```python
from build123d import *

# Parameters (mm, degrees)
SKETCH_1_R                         = 4
SKETCH_1_R_2                       = 1.5
SKETCH_1_R_3                       = 2
SM_BASE_FLANGE_1_DEPTH             = 2
SM_EDGE_FLANGE_1_STRIP_W           = 9.4732
SM_EDGE_FLANGE_1_STRIP_H           = 2
SM_EDGE_FLANGE_1_STRIP_CUT_DEPTH   = 9
SM_EDGE_FLANGE_1_STRIP_2_W         = 9.4732
SM_EDGE_FLANGE_1_STRIP_2_H         = 2
SM_EDGE_FLANGE_1_STRIP_CUT_2_DEPTH = 9
SM_EDGE_FLANGE_1_DEPTH             = 9
SM_EDGE_FLANGE_1_BEND_DEPTH        = 9
SM_EDGE_FLANGE_2_STRIP_W           = 9.4732
SM_EDGE_FLANGE_2_STRIP_H           = 2
SM_EDGE_FLANGE_2_STRIP_CUT_DEPTH   = 42
SM_EDGE_FLANGE_2_DEPTH             = 42
SKETCH_15_R                        = 1.5
CUT_EXTRUDE_1_DEPTH                = 10
SKETCH_16_R                        = 2
CUT_EXTRUDE_2_DEPTH                = 10
FILLET_1_R                         = 2


# Sheet-metal steps are written as plain solids
with BuildPart() as part:
    # Sketch 1 → 基体-法兰1 (new body)
    with BuildSketch(Plane.XY):
        Polygon((0, 0), (9, 0), (9, -6), (11, -6), (11, 4), (48, 4), (48, -6), (50, -6), (50, 0), (59, 0), (59, -25), (50.5, -25), (50.5, -33), (8.5, -33), (8.5, -25), (0, -25), align=None)
        with Locations((19, -8)):
            Circle(SKETCH_1_R, mode=Mode.SUBTRACT)
        with Locations((40, -8)):
            Circle(SKETCH_1_R, mode=Mode.SUBTRACT)
        with Locations((29.5, -19)):
            Circle(SKETCH_1_R, mode=Mode.SUBTRACT)
        with Locations((19, -1)):
            Circle(SKETCH_1_R_2, mode=Mode.SUBTRACT)
        with Locations((19, -15)):
            Circle(SKETCH_1_R_2, mode=Mode.SUBTRACT)
        with Locations((26, -8)):
            Circle(SKETCH_1_R_2, mode=Mode.SUBTRACT)
        with Locations((12, -8)):
            Circle(SKETCH_1_R_2, mode=Mode.SUBTRACT)
        with Locations(Location((33, -8, 0), (0, 0, 180))):
            Circle(SKETCH_1_R_2, mode=Mode.SUBTRACT)
        with Locations(Location((40, -15, 0), (0, 0, 180))):
            Circle(SKETCH_1_R_2, mode=Mode.SUBTRACT)
        with Locations(Location((47, -8, 0), (0, 0, 180))):
            Circle(SKETCH_1_R_2, mode=Mode.SUBTRACT)
        with Locations(Location((40, -1, 0), (0, 0, 180))):
            Circle(SKETCH_1_R_2, mode=Mode.SUBTRACT)
        with Locations((29.5, -12)):
            Circle(SKETCH_1_R_2, mode=Mode.SUBTRACT)
        with Locations((36.5, -19)):
            Circle(SKETCH_1_R_2, mode=Mode.SUBTRACT)
        with Locations((29.5, -26)):
            Circle(SKETCH_1_R_2, mode=Mode.SUBTRACT)
        with Locations((22.5, -19)):
            Circle(SKETCH_1_R_2, mode=Mode.SUBTRACT)
        with Locations((54, -9)):
            Circle(SKETCH_1_R_3, mode=Mode.SUBTRACT)
        with Locations((54, -19)):
            Circle(SKETCH_1_R_3, mode=Mode.SUBTRACT)
        with Locations((5, -19)):
            Circle(SKETCH_1_R_3, mode=Mode.SUBTRACT)
        with Locations((5, -9)):
            Circle(SKETCH_1_R_3, mode=Mode.SUBTRACT)
    extrude(amount=-SM_BASE_FLANGE_1_DEPTH)

    # 边线-法兰1 strip (across the edge) → 边线-法兰1 strip cut (cut)
    with BuildSketch(Plane(origin=(59, 0, 0), x_dir=(0, -1, 0), z_dir=(-1, 0, 0))):
        with Locations((-2, -1)):
            Rectangle(SM_EDGE_FLANGE_1_STRIP_W, SM_EDGE_FLANGE_1_STRIP_H)
    extrude(amount=SM_EDGE_FLANGE_1_STRIP_CUT_DEPTH, mode=Mode.SUBTRACT)

    # 边线-法兰1 strip 2 (across the edge) → 边线-法兰1 strip cut 2 (cut)
    with BuildSketch(Plane(origin=(9, 0, 0), x_dir=(0, -1, 0), z_dir=(-1, 0, 0))):
        with Locations((-2, -1)):
            Rectangle(SM_EDGE_FLANGE_1_STRIP_2_W, SM_EDGE_FLANGE_1_STRIP_2_H)
    extrude(amount=SM_EDGE_FLANGE_1_STRIP_CUT_2_DEPTH, mode=Mode.SUBTRACT)

    # 边线-法兰1 section (across the edge) → 边线-法兰1 (add)
    with BuildSketch(Plane(origin=(59, 0, 0), x_dir=(0, -1, 0), z_dir=(-1, 0, 0))):
        with BuildLine():
            Line((0, 0.7366), (0, 23))
            Line((0, 23), (2, 23))
            Line((2, 23), (2, 0.7366))
            ThreePointArc((2, 0.7366), (2.215745145, 0.215745145), (2.7366, 0))
            Line((2.7366, 0), (2.7366, -2))
            ThreePointArc((2.7366, -2), (0.801531583, -1.198468417), (0, 0.7366))
        make_face()
    extrude(amount=SM_EDGE_FLANGE_1_DEPTH)

    # 边线-法兰1 section 2 (across the edge) → 边线-法兰1 bend (add)
    with BuildSketch(Plane(origin=(9, 0, 0), x_dir=(0, -1, 0), z_dir=(-1, 0, 0))):
        with BuildLine():
            Line((0, 0.7366), (0, 23))
            Line((0, 23), (2, 23))
            Line((2, 23), (2, 0.7366))
            ThreePointArc((2, 0.7366), (2.215745145, 0.215745145), (2.7366, 0))
            Line((2.7366, 0), (2.7366, -2))
            ThreePointArc((2.7366, -2), (0.801531583, -1.198468417), (0, 0.7366))
        make_face()
    extrude(amount=SM_EDGE_FLANGE_1_BEND_DEPTH)

    # 边线-法兰2 strip (across the edge) → 边线-法兰2 strip cut (cut)
    with BuildSketch(Plane(origin=(8.5, -33, 0), x_dir=(0, 1, 0), z_dir=(1, 0, 0))):
        with Locations((-2, -1)):
            Rectangle(SM_EDGE_FLANGE_2_STRIP_W, SM_EDGE_FLANGE_2_STRIP_H)
    extrude(amount=SM_EDGE_FLANGE_2_STRIP_CUT_DEPTH, mode=Mode.SUBTRACT)

    # 边线-法兰2 section (across the edge) → 边线-法兰2 (add)
    with BuildSketch(Plane(origin=(8.5, -33, 0), x_dir=(0, 1, 0), z_dir=(1, 0, 0))):
        with BuildLine():
            Line((0, 0.7366), (0, 23))
            Line((0, 23), (2, 23))
            Line((2, 23), (2, 0.7366))
            ThreePointArc((2, 0.7366), (2.215745145, 0.215745145), (2.7366, 0))
            Line((2.7366, 0), (2.7366, -2))
            ThreePointArc((2.7366, -2), (0.801531583, -1.198468417), (0, 0.7366))
        make_face()
    extrude(amount=SM_EDGE_FLANGE_2_DEPTH)

    # 草图15 → 切除-拉伸1 (cut)
    with BuildSketch(Plane.XZ.offset(33)):
        with Locations(Location((47, 11.8683, 0), (0, 0, 270))):
            Circle(SKETCH_15_R)
        with Locations(Location((40, 11.8683, 0), (0, 0, 270))):
            Circle(SKETCH_15_R)
        with Locations(Location((33, 11.8683, 0), (0, 0, 270))):
            Circle(SKETCH_15_R)
        with Locations(Location((40, 4.8683, 0), (0, 0, 270))):
            Circle(SKETCH_15_R)
        with Locations(Location((40, 18.8683, 0), (0, 0, 270))):
            Circle(SKETCH_15_R)
        with Locations(Location((12, 11.8683, 0), (0, 0, 270))):
            Circle(SKETCH_15_R)
        with Locations(Location((19, 18.8683, 0), (0, 0, 270))):
            Circle(SKETCH_15_R)
        with Locations(Location((26, 11.8683, 0), (0, 0, 270))):
            Circle(SKETCH_15_R)
        with Locations(Location((19, 4.8683, 0), (0, 0, 270))):
            Circle(SKETCH_15_R)
        with Locations(Location((19, 11.8683, 0), (0, 0, 270))):
            Circle(SKETCH_15_R)
    extrude(amount=-CUT_EXTRUDE_1_DEPTH, mode=Mode.SUBTRACT)

    # 草图16 → 切除-拉伸2 (cut)
    with BuildSketch(Plane(origin=(0, 0, 0), x_dir=(1, 0, 0), z_dir=(0, 1, 0))):
        with Locations(Location((53.5, -17, 0), (0, 0, 270))):
            Circle(SKETCH_16_R)
        with Locations(Location((53.5, -7, 0), (0, 0, 270))):
            Circle(SKETCH_16_R)
        with Locations(Location((5.5, -17, 0), (0, 0, 90))):
            Circle(SKETCH_16_R)
        with Locations(Location((5.5, -7, 0), (0, 0, 90))):
            Circle(SKETCH_16_R)
    extrude(amount=-CUT_EXTRUDE_2_DEPTH, mode=Mode.SUBTRACT)

    # 圆角1
    fillet_1_edges = [part.edges().sort_by_distance(p)[0] for p in [
        (59, -1, 23),
        (50, -1, 23),
        (9, -1, 23),
        (0, -1, 23),
    ]]
    fillet(fillet_1_edges, radius=FILLET_1_R)


solid = part.part
```
The listing builds one solid part. Answer for the finished solid, in the listing's coordinates (mm). A direction names the side the tool comes from. Round coordinates to 2 decimals unless told otherwise and drop trailing zeros. Write each loop counter-clockwise with the first axis right and the second up, starting at its lowest first coordinate (ties: lowest second). Pieces come first, ordered by that corner, then holes. Notation, with made-up numbers: (15.5, 19) -> (48.5, 19) arc R30 ccw to (48.5, 52) -> close; hole circle Ø10 at (-30, 75.25). An arc over 180 degrees is marked (long way). Answer as a JSON object with one key per item and string values. Group by question number.
Q1. Section D-D (y = -19) is taken. Write down the section's boundary in (x, z).
Q2. Each of these flat-tipped pins is pushed along its axis until it touches: pin 1 Ø1 at (x, z) = (10, -1) entering from +Y; pin 2 Ø6.5 at (x, z) = (53.5, 7) entering from +Y; pin 3 Ø2.5 at (x, z) = (47, 11.87) entering from +Y; pin 4 Ø3.5 at (x, z) = (40, 4.87) entering from +Y. Where does it stop, or does it pass through?
Q3. Determine the mould class of faces 6 (the face through (17.5, -14.93, -0.99)), 7 (the face through (54.563, -0.823, -1.22)), 8 (the face through (11.675, -9.464, -0.986)), 9 (the face through (38.536, -32.014, 12.193)) for opening direction Y: pulls with the +Y half, pulls with the -Y half, needs draft (parallel to the pull), parting line crosses it, or undercut.
Q4. Which of the six approach directions +Z, -Z, +X, -X, +Y, -Y give full straight-line access (tool end or side, diameter ignored) to faces 1 (the face through (50, -1.7, 7.1)), 2 (the face through (4, -25, -1)), 3 (the face through (5, -2, 12)), 4 (the face through (50.57, -1.01, 22.4)), 5 (the face through (0, -8, -1))?
Q5. Section C-C (x = 19) is taken. Count the separate pieces of the cut face and the enclosed holes in it, plus the area to 3 significant figures.
Q6. Section B-B (x = 47) is taken. Write down the section's boundary in (y, z).
Q7. Straight lines are drawn through the part: line 1 along X through (y, z) = (-1.35, 17); line 2 along Y through (x, z) = (29.5, -1.3); line 3 along Y through (x, z) = (14, 13.25). For each, find the intervals that lie inside material, in ascending order.
Q8. Section A-A (z = 2.5) is taken. Write down the section's boundary in (x, y).
Check values:
{
 "1": {"outline": "(0, -2) -> (3, -2) -> (3, 0) -> (0, 0) -> close; (7, -2) -> (21, -2) -> (21, 0) -> (7, 0) -> close; (24, -2) -> (25.5, -2) -> (25.5, 0) -> (24, 0) -> close; (33.5, -2) -> (35, -2) -> (35, 0) -> (33.5, 0) -> close; (38, -2) -> (52, -2) -> (52, 0) -> (38, 0) -> close; (56, -2) -> (59, -2) -> (59, 0) -> (56, 0) -> close"},
 "2": {"pin 1": "y = -6", "pin 2": "y = 0", "pin 3": "through", "pin 4": "y = -31"},
 "3": {"face 6": "undercut", "face 7": "pulls with the +Y half", "face 8": "undercut", "face 9": "needs draft"},
 "4": {"face 1": "+Z, -Z, +Y", "face 2": "+Z, -Z, -X, -Y", "face 3": "+Z, +X, -X", "face 4": "+Z, +Y", "face 5": "+Z, -Z, -X, +Y, -Y"},
 "5": {"separate pieces": "7", "enclosed holes": "0", "area": "72.5 mm^2"},
 "6": {"outline": "(-33, 0.74) arc R2.74 ccw to (-30.26, -2) -> (-9.5, -2) -> (-9.5, 0) -> (-30.26, 0) arc R0.74 cw to (-31, 0.74) -> (-31, 10.37) -> (-33, 10.37) -> close; (-33, 13.37) -> (-31, 13.37) -> (-31, 23) -> (-33, 23) -> close; (-6.5, -2) -> (4, -2) -> (4, 0) -> (-6.5, 0) -> close"},
 "7": {"line 1": "0 to 3.5, 7.5 to 9, 50 to 51.5, 55.5 to 59", "line 2": "-32.09 to -27.5, -24.5 to -23, -15 to -13.5, -10.5 to 4", "line 3": "-33 to -31"},
 "8": {"outline": "(0, -2) -> (9, -2) -> (9, 0) -> (0, 0) -> close; (8.5, -33) -> (50.5, -33) -> (50.5, -31) -> (8.5, -31) -> close; (50, -2) -> (59, -2) -> (59, 0) -> (50, 0) -> close"}
}
